from build123d import *

# Parameters (mm, degrees)
SKETCH1_R           = 75
BOSS_EXTRUDE1_DEPTH = 2.5
SKETCH2_R           = 1.75
CUT_EXTRUDE1_DEPTH  = 107.09547587
SKETCH3_R           = 1.75
CUT_EXTRUDE2_DEPTH  = 107.09547587


with BuildPart() as part:
    # Sketch1 → Boss-Extrude1 (new body)
    with BuildSketch(Plane.XY):
        Circle(SKETCH1_R)
    extrude(amount=BOSS_EXTRUDE1_DEPTH)

    # Sketch2 → Cut-Extrude1 (cut, through all)
    with BuildSketch(Plane(origin=(0, 0, 0), x_dir=(-1, 0, 0), z_dir=(0, 0, -1))):
        with Locations((-50, 15)):
            Circle(SKETCH2_R)
        with Locations((-50, -15)):
            Circle(SKETCH2_R)
        with Locations((-15, -50)):
            Circle(SKETCH2_R)
        with Locations((15, -50)):
            Circle(SKETCH2_R)
        with Locations((50, -15)):
            Circle(SKETCH2_R)
        with Locations((50, 15)):
            Circle(SKETCH2_R)
        with Locations((-15, 50)):
            Circle(SKETCH2_R)
        with Locations((15, 50)):
            Circle(SKETCH2_R)
    extrude(amount=-CUT_EXTRUDE1_DEPTH, mode=Mode.SUBTRACT)

    # Sketch3 → Cut-Extrude2 (cut, through all)
    with BuildSketch(Plane(origin=(0, 0, 0), x_dir=(-1, 0, 0), z_dir=(0, 0, -1))):
        Circle(SKETCH3_R)
    extrude(amount=-CUT_EXTRUDE2_DEPTH, mode=Mode.SUBTRACT)


solid = part.part
Source: CAD feature listing. Evaluate the final solid. Frame: model axes, mm. Coordinates: 2 decimals unless noted, no trailing zeros. Loops run counter-clockwise (first coordinate to the right, second up) from the corner with the lowest first, then second, coordinate; pieces in that order, holes last. Notation, with made-up numbers: M 47,15 L 86,15 A27 ccw 86,40 Z; hole C 13,70.5 d4. An arc over 180 degrees is marked long. Answer in a Markdown table with one row per item.
Q1. Section A-A on z = 1. State how many separate pieces and enclosed holes the cut face has, plus the area to 3 significant figures.
Answers below:
| item | result |
|---|---|
| separate pieces | 1 |
| enclosed holes | 9 |
| area | 17,600 mm^2 |
Q2. Ray query, probe 1 along Y at (x, z) = (-15, 0.85); probe 2 along Y at (x, z) = (0, 0.75); probe 3 along Y at (x, z) = (50.5, 0.7). Return the intervals inside material, ascending. Write a range as from..to.
Answers below:
| item | result |
|---|---|
| probe 1 | y = -73.48..-51.75, -48.25..48.25, 51.75..73.48 |
| probe 2 | y = -75..-1.75, 1.75..75 |
| probe 3 | y = -55.45..-16.68, -13.32..13.32, 16.68..55.45 |
Q3. Section B-B on x = 0. Return the cut outline in (y, z), plus the area to 3 significant figures.
Answers below:
| item | result |
|---|---|
| outline | M -75,0 L -1.75,0 L -1.75,2.5 L -75,2.5 Z; M 1.75,0 L 75,0 L 75,2.5 L 1.75,2.5 Z |
| area | 366 mm^2 |
Q4. Draft query along Y for faces 1 (the cylindrical face through (-14.62, 48.29, 1.23)), 2 (the cylindrical face through (-9.764, 74.362, 1.232)), 3 (the flat face through (-1, -16, 2.5)). Return one class per face: pulls with the +Y half, pulls with the -Y half, needs draft (parallel to the pull), parting line crosses it, or undercut.
Answers below:
| item | result |
|---|---|
| face 1 | undercut |
| face 2 | parting line crosses it |
| face 3 | needs draft |
Q5. Section D-D on y = 15. Return the cut outline in (x, z).
Answers below:
| item | result |
|---|---|
| outline | M -73.48,0 L -51.75,0 L -51.75,2.5 L -73.48,2.5 Z; M -48.25,0 L 48.25,0 L 48.25,2.5 L -48.25,2.5 Z; M 51.75,0 L 73.48,0 L 73.48,2.5 L 51.75,2.5 Z |
Q6. First-contact query: pin 1 (3 mm diameter, centred on x = -15, y = -50, fed in from +Z). Flat tip, straight axial feed; report the tip coordinate or a pass-through.
Answers below:
| item | result |
|---|---|
| pin 1 | passes through |
